The listing builds one solid part. Answer for the finished solid, in the listing's coordinates (mm). Round coordinates to 2 decimals unless told otherwise and drop trailing zeros. Write each loop counter-clockwise with the first axis right and the second up, starting at its lowest first coordinate (ties: lowest second). Pieces come first, ordered by that corner, then holes.
(1) A cutting plane is placed at B-B, the plane z = 1.4. Give the number of separate pieces and of enclosed holes in the cut face, and give its area (3 significant figures).
(2) A cutting plane is placed at A-A, the plane y = -37. Give the vertices of the cut face in (x, z).
(3) A cutting plane is placed at C-C, the plane x = -54.5. Give the vertices of the cut face in (y, z).
(4) Each of these flat-tipped pins is pushed along its axis until it touches: pin 1 Ø1.4 at (x, z) = (18.5, 2.5) entering from +Y; pin 2 Ø3 at (y, z) = (-30.5, 3) entering from +X; pin 3 Ø1.5 at (y, z) = (2.5, 3.5) entering from -X. Where does it stop, or does it pass through?
(5) Find the intervals of material crossed by probe 1 along Y at (x, z) = (0, 3.5); probe 2 along X at (y, z) = (-17, 3.4); probe 3 along Y at (x, z) = (-8.85, 1.4), in increasing order.
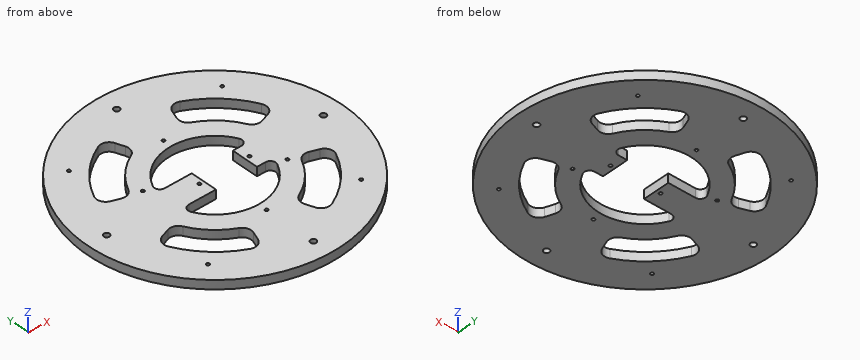
Autodesk Inventor part; units mm, degrees
ref_plane "YZ Plane" through (0, 0, 0) normal (1, 0, 0) x (0, 1, 0)
ref_plane "XZ Plane" through (0, 0, 0) normal (0, 1, 0) x (-1, 0, 0)
ref_plane "XY Plane" through (0, 0, 0) normal (0, 0, 1) x (1, 0, 0)
sketch "스케치1" plane through (0, 0, 0) normal (0, 0, 1) x (1, 0, 0)
  circle A0 centre (0, 0) radius 27
  circle A1 centre (0, 0) radius 71.7255
  dimension "d0" = 54
  dimension "d1" = 143.451
extrude "돌출1" add sketch "스케치1" along normal blind 5
sketch "스케치2" plane through (0, 0, 5) normal (0, 0, 1) x (1, 0, 0)
  circle A0 centre (0, 0) radius 32
  circle A1 centre (0, 32) radius 0.85
  circle A2 centre (0, -32) radius 0.85
  line L0 (0, 0) -> (0, -32) construction
  line L1 (0, 0) -> (29.5641, -12.2459) construction
  circle A3 centre (29.5641, -12.2459) radius 0.85
  line L2 (0, 0) -> (-29.5641, 12.2459) construction
  circle A4 centre (-29.5641, 12.2459) radius 0.85
  dimension "d4" = 64
  dimension "d5" = 1.7
  dimension "d6" = 1.7
  dimension "d7" = 1.7
  dimension "d8" = 67.5
  dimension "d9" = 1.7
extrude "돌출2" cut sketch "스케치2" against normal blind 10 contours A1 A0 | A0 A1 | A3 A0 | A0 A3 | A4 A0 | A0 A4 | A2 A0 | A0 A2
sketch "스케치3" plane through (0, 0, 0) normal (0, 0, -1) x (-1, 0, 0)
  circle A0 centre (0, 0) radius 61
  circle A1 centre (61, 0) radius 1.6
  circle A2 centre (0, 61) radius 1.6
  circle A3 centre (-61, 0) radius 1.6
  circle A4 centre (0, -61) radius 1.6
  dimension "d12" = 122
  dimension "d13" = 3.2
  dimension "d16" = 360
extrude "돌출3" cut sketch "스케치3" against normal blind 10 contours A0 A1 | A0 A1 | A2 A0 | A0 A2 | A4 A0 | A0 A4 | A3 A0 | A0 A3
sketch "스케치4" plane through (0, 0, 0) normal (0, 0, -1) x (-1, 0, 0)
  circle A0 centre (0, 0) radius 2.5
  line L0 (0, 0) -> (8.85, 0)
  line L1 (0, 0) -> (-19.35, 0)
  circle A1 centre (8.85, 0) radius 0.85
  circle A2 centre (-19.35, 0) radius 0.85
  line L2 (-29.4038, 7.5) -> (29.4038, 7.5)
  line L3 (29.4038, 7.5) -> (29.4038, -7.5)
  line L4 (29.4038, -7.5) -> (-29.4038, -7.5)
  line L5 (-29.4038, -7.5) -> (-29.4038, 7.5)
  line L6 (-29.4038, 7.5) -> (29.4038, -7.5) construction
  line L7 (29.4038, 7.5) -> (-29.4038, -7.5) construction
  line L8 (-5, -7.5) -> (6.3, -7.5)
  line L9 (10.85, 7.5) -> (6.3, 7.5)
  line L10 (6.3, 7.5) -> (6.3, -7.5)
  line L11 (6.3, -7.5) -> (10.85, -7.5)
  line L12 (10.85, -7.5) -> (10.85, 7.5) construction
  line L13 (-16.8, 7.5) -> (-21.35, 7.5)
  line L14 (-21.35, 7.5) -> (-21.35, -7.5) construction
  line L15 (-21.35, -7.5) -> (-16.8, -7.5)
  line L16 (-16.8, -7.5) -> (-16.8, 7.5)
  point P0 (-16.8, -7.5)
  point P1 (6.3, -7.5)
  point P2 (6.3, 7.5)
  dimension "d20" = 5
  dimension "d21" = 8.85
  dimension "d22" = 19.35
  dimension "d23" = 1.7
  dimension "d24" = 1.7
  dimension "d25" = 15
  dimension "d29" = 16.8
  dimension "d30" = 21.35
  dimension "d31" = 10.85
  dimension "d32" = 6.3
extrude "돌출4" add sketch "스케치4" against normal blind 5 contours L10 L2 L3 L4 | L16 L4 L5 L2
fillet "모깎기1" radius 3 4 edges at (25.9374, -7.5, 2.5) (-25.9374, -7.5, 2.5) (-25.9374, 7.5, 2.5) (25.9374, 7.5, 2.5)
sketch "스케치6" plane through (0, 0, 0) normal (0, 0, -1) x (-1, 0, 0)
  circle A0 centre (0, 0) radius 52.5
  circle A1 centre (0, 0) radius 37.5
  line L0 (0, 0) -> (0, -83.3327)
  line L1 (0, 0) -> (22.8876, -62.8832)
  line L2 (0, 0) -> (58.8648, -21.425)
  point P0 (49.3339, -17.9561)
  point P1 (35.2385, -12.8258)
  point P2 (12.8258, -35.2385)
  point P3 (17.9561, -49.3339)
  dimension "d34" = 105
  dimension "d35" = 75
  dimension "d36" = 20
  dimension "d37" = 50
extrude "돌출5" cut sketch "스케치6" against normal blind 5 contours A0 L1 A1 L2
fillet "모깎기2" radius 5 4 edges at (-35.2385, -12.8258, 2.5) (-49.3339, -17.9561, 2.5) (-17.9561, -49.3339, 2.5) (-12.8258, -35.2385, 2.5)
pattern_circular "원형 패턴1" count 4 over 360 about axis through (0, 0, 0) along (0, 0, 1) of "돌출5", "모깎기2"
sketch "스케치7" plane through (0, 0, 0) normal (0, 0, -1) x (-1, 0, 0)
  circle A0 centre (0, -61) radius 1.6
  circle A1 centre (0, 0) radius 61 construction
  circle A2 centre (43.1335, -43.1335) radius 0.85
  line L0 (43.1335, -43.1335) -> (0, 0) construction
  line L1 (0, 0) -> (0, -16.1996)
  circle A3 centre (43.1335, 43.1335) radius 0.85
  circle A4 centre (-43.1335, 43.1335) radius 0.85
  circle A5 centre (-43.1335, -43.1335) radius 0.85
  dimension "d44" = 1.7
  dimension "d45" = 45
  dimension "d48" = 360
extrude "돌출6" cut sketch "스케치7" against normal blind 5 contours A2 | A3 | A4 | A5
properties part number "아크릴 빛번짐"
Solutions:
1. separate pieces: 1
1. enclosed holes: 19
1. area: 12,000 mm2
2. outline: (-61.45, 0) - (-37.25, 0) - (-37.25, 5) - (-61.45, 5) - close; (-14.22, 0) - (14.22, 0) - (14.22, 5) - (-14.22, 5) - close; (37.25, 0) - (61.45, 0) - (61.45, 5) - (37.25, 5) - close
3. outline: (-46.63, 0) - (46.63, 0) - (46.63, 5) - (-46.63, 5) - close
4. pin 1: stops at y = 69.48
4. pin 2: stops at x = 65.6
4. pin 3: stops at x = -71.7
5. probe 1: y = -71.73 to -62.6, -59.4 to -32.85, -31.15 to -27, 27 to 31.15, 32.85 to 59.4, 62.6 to 71.73
5. probe 2: x = -69.68 to -45.86, -33.43 to -20.98, 20.98 to 33.43, 45.86 to 69.68
5. probe 3: y = -71.18 to -25.51, -7.5 to -0.85, 0.85 to 7.5, 25.51 to 71.18
